```python
from build123d import *

# Parameters (mm, degrees)
SKETCH_2_R           = 1.795
EXTRUDE_1_DEPTH      = 1.25
EXTRUDE_2_DEPTH      = 5.1
EXTRUDE_2_DEPTH_BACK = 5.1
SKETCH_1_R           = 1.795


with BuildPart() as part:
    # Sketch 2 → Extrude 1 (new body)
    with BuildSketch(Plane.XY.offset(5)):
        with BuildLine():
            ThreePointArc((3.175, -8.746386407), (11.3, -4.948772024), (3.175, -1.151157641))
            ThreePointArc((3.175, -1.151157641), (0, -2.303543258), (-3.175, -1.151157641))
            ThreePointArc((-3.175, -1.151157641), (-11.3, -4.948772024), (-3.175, -8.746386407))
            ThreePointArc((-3.175, -8.746386407), (0, -7.594000789), (3.175, -8.746386407))
        make_face()
        with Locations((6.35, -4.948772024)):
            Circle(SKETCH_2_R, mode=Mode.SUBTRACT)
        with Locations((-6.35, -4.948772024)):
            Circle(SKETCH_2_R, mode=Mode.SUBTRACT)
    extrude(amount=-EXTRUDE_1_DEPTH)


with BuildPart() as body_2:
    # Mirror 3: mirrored copy
    add(part.part.mirror(Plane.XY))


with BuildPart() as part_1:
    add(part.part)

    add(body_2.part)  # Extrude 2 merges body 2
    # Sketch 1 → Extrude 2 (add, two sides: drawn at the far end of the back side and taken through both)
    with BuildSketch(Plane.XY.offset(-EXTRUDE_2_DEPTH_BACK)):
        with Locations((6.35, -4.948772024)):
            Circle(SKETCH_1_R)
        with Locations((-6.35, -4.948772024)):
            Circle(SKETCH_1_R)
    extrude(amount=EXTRUDE_2_DEPTH + EXTRUDE_2_DEPTH_BACK)


solid = part_1.part
```
The model under review builds one solid part; all positions refer to its coordinate system, in mm. A direction names the side the tool comes from. Round coordinates to 2 decimals unless told otherwise and drop trailing zeros. Order: outer loops, then holes, each group sorted by start corner. A loop starts at its lowest first (then second) coordinate and runs counter-clockwise, first axis right, second up. Notation, with made-up numbers: M 21.25,48.25 L 57.25,48.25 A20 ccw 57.25,81.25 Z; hole C 42,87 d10. An arc over 180 degrees is marked long. Use a Markdown table: item, result.
1) Insertion check: pin 1 (6 mm diameter, centred on x = -3, z = 4, fed in from -Y); pin 2 (4 mm diameter, centred on x = 7.5, z = 0, fed in from +Y). Each pin has a flat end and moves straight along its axis. Give the tip position at first contact, or say it passes through.
Report:
| item | result |
|---|---|
| pin 1 | y = -9.89 |
| pin 2 | y = -3.15 |
2) Draft analysis for pull direction X (two halves, no side actions). For faces 4 (the face through (-6, -5, -5.1)), 5 (the face through (0, -5, 5)), 6 (the face through (5.96, -6.7, -0.05)), state which applies: released by +X, released by -X, zero draft, split by the parting line, or undercut.
Report:
| item | result |
|---|---|
| face 4 | zero draft |
| face 5 | undercut |
| face 6 | undercut |
3) Consider section A-A (x = -0.75). Write out the cut boundary in (y, z), then the cut area to 3 significant figures.
Report:
| item | result |
|---|---|
| outline | M -7.65,-5 L -2.25,-5 L -2.25,-3.75 L -7.65,-3.75 Z; M -7.65,3.75 L -2.25,3.75 L -2.25,5 L -7.65,5 Z |
| area | 13.5 mm^2 |
4) Tool access review of faces 1 (the face through (0, -5, -5)), 2 (the face through (0, -5, 3.75)), 3 (the face through (6, -5, -5.1)): name each direction out of +Z, -Z, +X, -X, +Y, -Y from which nothing blocks a thin tool from reaching the whole face with its end or side.
Report:
| item | result |
|---|---|
| face 1 | -Z |
| face 2 | none |
| face 3 | -Z, +X, -X, +Y, -Y |
5) Consider section C-C (y = -9). Write out the cut boundary in (x, z).
Report:
| item | result |
|---|---|
| outline | M -9.19,-5 L -3.51,-5 L -3.51,-3.75 L -9.19,-3.75 Z; M -9.19,3.75 L -3.51,3.75 L -3.51,5 L -9.19,5 Z; M 3.51,-5 L 9.19,-5 L 9.19,-3.75 L 3.51,-3.75 Z; M 3.51,3.75 L 9.19,3.75 L 9.19,5 L 3.51,5 Z |
6) Consider section B-B (x = -6.35). Write out the cut boundary in (y, z), then the cut area to 3 significant figures.
Report:
| item | result |
|---|---|
| outline | M -9.9,-5 L -6.74,-5 L -6.74,-5.1 L -3.15,-5.1 L -3.15,-5 L 0,-5 L 0,-3.75 L -3.15,-3.75 L -3.15,3.75 L 0,3.75 L 0,5 L -3.15,5 L -3.15,5.1 L -6.74,5.1 L -6.74,5 L -9.9,5 L -9.9,3.75 L -6.74,3.75 L -6.74,-3.75 L -9.9,-3.75 Z |
| area | 52.4 mm^2 |
7) Wall thickness on line 1 along Z through (x, y) = (1.5, -2.25); line 2 along X through (y, z) = (-4, 1.5); line 3 along X through (y, z) = (-8, 4.5): over which ranges is each line inside the solid? List them lowest first. Write a range as [from, to].
Report:
| item | result |
|---|---|
| line 1 | [-5, -3.75], [3.75, 5] |
| line 2 | [-7.87, -4.83], [4.83, 7.87] |
| line 3 | [-10.25, -1.96], [1.96, 10.25] |
